from build123d import *

# Parameters (mm, degrees)
SKETCH1_R              = 3.5
SKETCH1_R_2            = 2.25
BOSS_EXTRUDE1_DEPTH    = 2.7
SKETCH2_R              = 1.6
SKETCH2_R_2            = 1.5
BOSS_EXTRUDE2_DEPTH    = 1.8
BOSS_EXTRUDE3_DEPTH    = 3.9
FILLET1_R              = 10
CUT_EXTRUDE1_START     = -2
CUT_EXTRUDE1_OUTLINE_R = 1.6
CUT_EXTRUDE1_DEPTH     = 2
FILLET2_R              = 2


# Read off the part's stored shape, not the designer's step: Cut-Extrude1
with BuildPart() as part:
    # Sketch1 → Boss-Extrude1 (new body)
    with BuildSketch(Plane(origin=(0, 0, 0), x_dir=(1, 0, 0), z_dir=(0, 1, 0))):
        with Locations(Location((0, 0, 0), (0, 0, 90))):
            Circle(SKETCH1_R)
        with Locations(Location((0, 0, 0), (0, 0, 90))):
            Circle(SKETCH1_R_2, mode=Mode.SUBTRACT)
    extrude(amount=BOSS_EXTRUDE1_DEPTH)

    # Sketch2 → Boss-Extrude2 (add)
    with BuildSketch(Plane(origin=(0, 2.7, 0), x_dir=(1, 0, 0), z_dir=(0, 1, 0))):
        with BuildLine():
            Line((0, 3.9), (-30.1, 3.9))
            ThreePointArc((-30.1, 3.9), (-34, 0), (-30.1, -3.9))
            Line((-30.1, -3.9), (0, -3.9))
            ThreePointArc((0, -3.9), (3.9, 0), (0, 3.9))
        make_face()
        with Locations(Location((-30, 0, 0), (0, 0, 270))):
            Circle(SKETCH2_R, mode=Mode.SUBTRACT)
        with Locations(Location((0, 0, 0), (0, 0, 270))):
            Circle(SKETCH2_R_2, mode=Mode.SUBTRACT)
    extrude(amount=BOSS_EXTRUDE2_DEPTH)

    # Sketch3 → Boss-Extrude3 (add, symmetric)
    with BuildSketch(Plane.XY):
        Polygon((-25.4, 2.7), (-2.25, 2.7), (-2.25, 0), (-3.5, 0), (-25.4, 0), align=None)
        Polygon((-34, 0.7), (-25.4, 0.7), (-25.4, 2.7), (-28.4, 2.7), (-31.6, 2.7), (-34, 2.7), align=None)
    extrude(amount=BOSS_EXTRUDE3_DEPTH, both=True)

    # Fillet1
    # the kernel refuses this fillet: 10 mm, written as the material it adds along each edge
    with BuildSketch(Plane(origin=(-2.25, 2.7, -2.680951324), x_dir=(0.9469829588957737, 0, -0.3212837928701128), z_dir=(0, -1, 0))) as fillet1_piece_1:
        with BuildLine():
            CenterArc((6.165489318, -9.319153575), FILLET1_R, 111.264619874, 14.002057775)
            Line((0.391660582, -1.154418323), (0.276184008, -0.991123617))
            ThreePointArc((0.276184008, -0.991123617), (0.006433699, -0.64146592), (-0.189396592, -0.064256759))
            Line((-0.189396592, -0.064256759), (0.072535168, 0.186383071))
            ThreePointArc((0.072535168, 0.186383071), (1.269365448, -0.038296249), (2.466195727, 0.186383071))
            Line((2.466195727, 0.186383071), (2.538730895, 0))
        make_face()
    extrude(amount=2.7)
    with BuildSketch(Plane(origin=(-2.25, 2.7, 2.680951324), x_dir=(1.3741079680414238e-12, 0, 1.0), z_dir=(0, -1, 0))) as fillet1_piece_2:
        with BuildLine():
            CenterArc((10.805951419, -2.84452031), FILLET1_R, 163.473903362, 14.002057775)
            Line((0.815653091, -2.404134895), (0.615847125, -2.395327187))
            ThreePointArc((0.615847125, -2.395327187), (0.444092441, -1.189763484), (-0.153197218, -0.128571429))
            Line((-0.153197218, -0.128571429), (0, 0.2))
            ThreePointArc((0, 0.2), (0.609524338, 0.2), (1.027310621, 0.056890406))
            Line((1.027310621, 0.056890406), (1.219048676, 0))
        make_face()
    extrude(amount=2.7)

    # Cut-Extrude1 outline → Cut-Extrude1 (cut)
    with BuildSketch(Plane(origin=(0, 2.7, 0), x_dir=(1, 0, 0), z_dir=(0, 1, 0)).offset(CUT_EXTRUDE1_START)):
        with BuildLine():
            Line((-34, -3.9), (-30.1, -3.9))
            ThreePointArc((-30.1, -3.9), (-32.857716447, -2.757716447), (-34, 0))
            Line((-34, 0), (-34, -3.9))
        make_face()
        with BuildLine():
            Line((-34, 3.9), (-34, 0))
            ThreePointArc((-34, 0), (-32.857716447, 2.757716447), (-30.1, 3.9))
            Line((-30.1, 3.9), (-34, 3.9))
        make_face()
        with Locations((-30, 0)):
            Circle(CUT_EXTRUDE1_OUTLINE_R)
    extrude(amount=CUT_EXTRUDE1_DEPTH, mode=Mode.SUBTRACT)

    # Fillet2
    # the kernel refuses this fillet: 2 mm, written as the material it adds along each edge
    with BuildSketch(Plane(origin=(-25.4, 0.7, -3.9), x_dir=(-1, 0, 0), z_dir=(0, 0, 1))) as fillet2_piece_1:
        with BuildLine():
            CenterArc((1.519868415, 2), FILLET2_R, 220.541601874, 49.458398126)
            Line((0, 0.7), (-0.030397368, 0.674))
            ThreePointArc((-0.030397368, 0.674), (-0.04, 0.35), (-0.04, 0))
            Line((-0.04, 0), (0, -0.04))
            Line((0, -0.04), (1.519868415, -0.04))
            Line((1.519868415, -0.04), (1.519868415, 0))
        make_face()
    extrude(amount=7.8)


solid = part.part
Here's how the part is built. I have some questions about the finished solid (model axes, mm). A direction names the side the tool comes from. Give positions to 0.01 mm unless a question says otherwise; leave off trailing zeros. Write each loop counter-clockwise with the first axis right and the second up, starting at its lowest first coordinate (ties: lowest second). Pieces come first, ordered by that corner, then holes. Notation, with made-up numbers: (-38, 39) -> (3, 39) arc R18 ccw to (3, 45) -> close; hole circle Ø9 at (-1, -17). An arc over 180 degrees is marked (long way). Use one line per item in the form item = value. Start each with the question number.
1. If I drill on L1, parallel to Z at x = -30, y = 1.8; L2, parallel to X at y = 3.95, z = 0; L3, parallel to X at y = 1.45, z = -0.5, over which ranges is the centre line in solid material (lowest first)?
2. Imagine slicing it at C-C on z = -0.5. List the corners of the cut face in (x, y) for me.
3. Thinking about a two-plate mould opening in Z: for faces 1 (the face through (-2, 2.7, 0)), 2 (the face through (-26.07, 0.51, -0.05)), 3 (the face through (-15, 2, -3.9)), which applies, +Z half, -Z half, draft (parallel to the pull), parting line (faces both ways), or undercut?
4. On a 3-axis mill with a long thin cutter (end or side, diameter ignored), from which of +Z, -Z, +X, -X, +Y, -Y can I reach the whole of each face in a straight line? I mean faces 4 (the face through (3.5, 1.3, 0.1)), 5 (the face through (-31, 0.7, -2)), 6 (the face through (-0.676, 1.331, -2.146)). Say none if no direction works.
5. Imagine slicing it at A-A on y = 3.65. List the corners of the cut face in (x, z) for me.
6. Will these pins go through, and if not, where does the flat tip stop? pin 1 Ø1.5 at (y, z) = (1, -1.5) entering from +X; pin 2 Ø1 at (y, z) = (2.5, -2) entering from -X; pin 3 Ø1.5 at (y, z) = (1, 1) entering from -X.
7. Imagine slicing it at D-D on y = 1.2. List the corners of the cut face in (x, z) for me.
Entries:
q1.L1 = -3.9 to -1.6, 1.6 to 3.9
q1.L2 = -34 to -31.6, -28.4 to -1.5, 1.5 to 3.9
q1.L3 = -33.97 to -31.52, -28.48 to -2.19, 2.19 to 3.46
q2.outline = (-33.97, 0.7) -> (-31.52, 0.7) -> (-31.52, 4.5) -> (-33.97, 4.5) -> close; (-28.48, 0.7) -> (-26.92, 0.7) arc R2 cw to (-25.4, 0) -> (-2.19, 0) -> (-2.19, 2.7) -> (-1.41, 2.7) -> (-1.41, 4.5) -> (-28.48, 4.5) -> close; (1.41, 2.7) -> (2.19, 2.7) -> (2.19, 0) -> (3.46, 0) -> (3.46, 2.7) -> (3.87, 2.7) -> (3.87, 4.5) -> (1.41, 4.5) -> close
q3.face_1 = undercut
q3.face_2 = draft
q3.face_3 = -Z half
q4.face_4 = +X, -Y
q4.face_5 = +Z, -Z, -X, -Y
q4.face_6 = -Y
q5.outline = (-30.1, -3.9) -> (0, -3.9) arc R3.9 ccw to (0, 3.9) -> (-30.1, 3.9) arc R3.9 ccw to start; hole circle Ø3.2 at (-30, 0); hole circle Ø3 at (0, 0)
q6.pin_1 = 3.42
q6.pin_2 = -33.7
q6.pin_3 = -33.99
q7.outline = (-30.1, -3.9) -> (-2.25, -3.9) arc R10 cw to (0.15, -3.5) arc R3.5 ccw to (0.15, 3.5) arc R10 cw to (-2.25, 3.9) -> (-30.1, 3.9) arc R3.9 ccw to start; hole circle Ø3.2 at (-30, 0); hole circle Ø4.5 at (0, 0)
